Part model, mm, in its own coordinate system. A direction names the side the tool comes from. Round coordinates to 2 decimals unless told otherwise and drop trailing zeros. Loops run counter-clockwise (first coordinate to the right, second up) from the corner with the lowest first, then second, coordinate; pieces in that order, holes last. Notation, with made-up numbers: (52, 88) -> (106, 88) arc R14 ccw to (106, 104) -> close; hole circle Ø4 at (30, 3). An arc over 180 degrees is marked (long way). Use a Markdown table: item, result. Add a question column.
Item 1: Probe line 1 (X direction, y = -0.65, z = 105.5); line 2 (Z direction, x = -8, y = -0.2). List the from-to ranges inside material, lowest first. Write a range as [from, to].
Item 2: Flat gauge pin, fed straight in: pin 1 (3 mm diameter, centred on x = -0.5, z = 126, fed in from +Y). Where does the tip first touch, or does it go through?
Item 3: Cut at A-A, the plane z = 84.5. List the corners of the cut face in (x, y), plus the area to 3 significant figures.
Item 4: Two-plate mould, pull along Z, no slides. Class faces 1 (the face through (-44.45, -2, 75)), 2 (the face through (25.504, -2, 78)), 3 (the face through (-6, -2, 152.4)), 4 (the face through (28.749, -1.623, 15.582)): pulls with the +Z half, pulls with the -Z half, needs draft (parallel to the pull), parting line crosses it, or undercut.
Item 5: Cut at B-B, the plane y = -0.95. State how many separate pieces and enclosed holes the cut face has, plus the area to 3 significant figures.
Item 6: Which spindle directions (+Z, -Z, +X, -X, +Y, -Y) get a long thin tool onto all of the face, cutting with end or side? Do faces 5 (the face through (-41.91, -2, 79)), 6 (the face through (-6, -3.2, 75)). Say none if no direction does.
```python
from build123d import *

# Parameters (mm, degrees)
SKETCH2_W           = 78.8444702
SKETCH2_H           = 3.2004
BOSS_EXTRUDE1_DEPTH = 152.4
SKETCH3_R           = 1.1303
SKETCH3_W           = 12.7
SKETCH3_H           = 22.86
CUT_EXTRUDE1_DEPTH  = 159.782256755
FILLET1_R           = 2.54


with BuildPart() as part:
    # Sketch2 → Boss-Extrude1 (new body)
    with BuildSketch(Plane.XY):
        with Locations((-5.0277649, -1.6002)):
            Rectangle(SKETCH2_W, SKETCH2_H)
    extrude(amount=BOSS_EXTRUDE1_DEPTH)

    # Sketch3 → Cut-Extrude1 (cut, through all)
    with BuildSketch(Plane.XZ.offset(3.2004)):
        with Locations(Location((-40.132, 148.082, 0), (0, 0, 270))):
            Circle(SKETCH3_R)
        with Locations(Location((30.0764702, 148.082, 0), (0, 0, 270))):
            Circle(SKETCH3_R)
        with Locations(Location((-40.132, 4.318, 0), (0, 0, 270))):
            Circle(SKETCH3_R)
        with Locations(Location((30.0764702, 4.318, 0), (0, 0, 270))):
            Circle(SKETCH3_R)
        with Locations(Location((-5.0277649, 30.425887591, 0), (0, 0, 270))):
            Circle(SKETCH3_R)
        with Locations(Location((-5.0277649, 2.765287591, 0), (0, 0, 270))):
            Circle(SKETCH3_R)
        with BuildLine():
            Line((-41.91, 19.097412352), (-41.91, 139.804041398))
            ThreePointArc((-41.91, 139.804041398), (-39.076175505, 142.637865893), (-36.24235101, 139.804041398))
            Line((-36.24235101, 139.804041398), (-36.24235101, 19.097412352))
            ThreePointArc((-36.24235101, 19.097412352), (-39.076175505, 16.263587857), (-41.91, 19.097412352))
        make_face()
        with BuildLine():
            Line((25.5044702, 18.756236847), (25.5044702, 139.462865893))
            ThreePointArc((25.5044702, 139.462865893), (28.6794702, 142.637865893), (31.8544702, 139.462865893))
            Line((31.8544702, 139.462865893), (31.8544702, 18.756236847))
            ThreePointArc((31.8544702, 18.756236847), (28.6794702, 15.581236847), (25.5044702, 18.756236847))
        make_face()
        with Locations((-5.0277649, 16.595587591)):
            Rectangle(SKETCH3_W, SKETCH3_H)
    extrude(amount=-CUT_EXTRUDE1_DEPTH, mode=Mode.SUBTRACT)

    # Fillet1
    fillet1_edges = [part.edges().sort_by_distance(p)[0] for p in [
        (34.3944702, -1.6002, 152.4),
        (-44.45, -1.6002, 152.4),
        (34.3944702, -1.6002, 0),
        (-44.45, -1.6002, 0),
    ]]
    fillet(fillet1_edges, radius=FILLET1_R)


solid = part.part
```
A:
| question | item | result |
|---|---|---|
| 1 | line 1 | x = [-44.45, -41.91], [-36.24, 25.5], [31.85, 34.39] |
| 1 | line 2 | z = [0, 5.17], [28.03, 152.4] |
| 2 | pin 1 | stops at y = 0 |
| 3 | outline | (-44.45, -3.2) -> (-41.91, -3.2) -> (-41.91, 0) -> (-44.45, 0) -> close; (-36.24, -3.2) -> (25.5, -3.2) -> (25.5, 0) -> (-36.24, 0) -> close; (31.85, -3.2) -> (34.39, -3.2) -> (34.39, 0) -> (31.85, 0) -> close |
| 3 | area | 214 mm^2 |
| 4 | face 1 | needs draft |
| 4 | face 2 | undercut |
| 4 | face 3 | pulls with the +Z half |
| 4 | face 4 | undercut |
| 5 | separate pieces | 1 |
| 5 | enclosed holes | 9 |
| 5 | area | 10,200 mm^2 |
| 6 | face 5 | +Y, -Y |
| 6 | face 6 | +Z, -Z, +X, -X, -Y |
